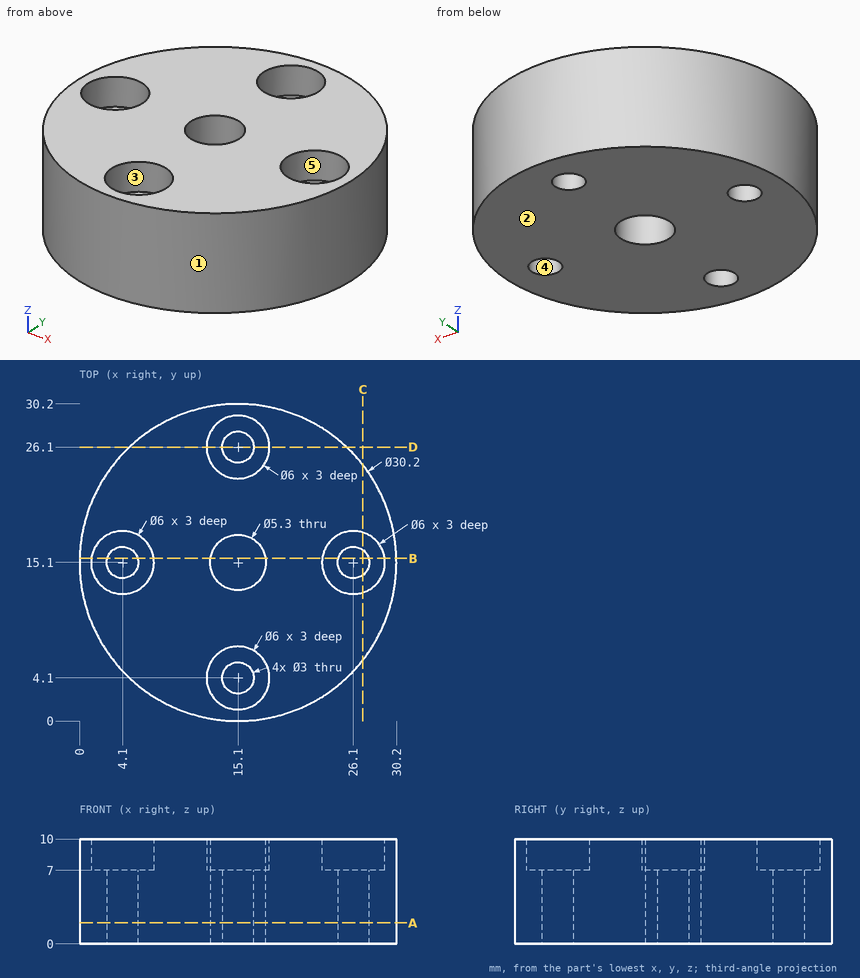
Study the drawing (mm; zero at the part's minimum x, y, z) and answer. A direction names the side the tool comes from. Round coordinates to 2 decimals unless told otherwise and drop trailing zeros. Loops run counter-clockwise (first coordinate to the right, second up) from the corner with the lowest first, then second, coordinate; pieces in that order, holes last. Notation, with made-up numbers: M 84,1.5 L 112,1.5 A21 cw 112,7.5 Z; hole C 65,86.25 d4. An arc over 180 degrees is marked long. One line per question, with ' | ' between items.
Q1. Find section B-B, the plane y = 15.5. Give the vertices of the cut face in (x, z).
Conclusion:
outline: M 0.01,0 L 2.65,0 L 2.65,7 L 1.13,7 L 1.13,10 L 0.01,10 Z; M 5.55,0 L 12.48,0 L 12.48,10 L 7.07,10 L 7.07,7 L 5.55,7 Z; M 17.72,0 L 24.65,0 L 24.65,7 L 23.13,7 L 23.13,10 L 17.72,10 Z; M 27.55,0 L 30.19,0 L 30.19,10 L 29.07,10 L 29.07,7 L 27.55,7 Z
Q2. Find section D-D, the plane y = 26.1. Give the vertices of the cut face in (x, z).
Conclusion:
outline: M 4.76,0 L 13.6,0 L 13.6,7 L 12.1,7 L 12.1,10 L 4.76,10 Z; M 16.6,0 L 25.44,0 L 25.44,10 L 18.1,10 L 18.1,7 L 16.6,7 Z
Q3. A tool of negligible diameter and unlimited length cuts with its end or side. For the marked faces 4 and 5, from which of +Z, -Z, +X, -X, +Y, -Y can it reach the whole face along a straight path? Write none if from no direction.
Conclusion:
face 4: +Z, -Z | face 5: +Z
Q4. Consider line 1 along Y through (x, z) = (15.1, 1.5); line 2 along Z through (x, y) = (13.5, 2); line 3 along Y through (x, z) = (25, 4.5). Determine where each line is inside the solid, lowest interval first. Write a range as from..to.
Conclusion:
line 1: y = 0..2.6, 5.6..12.45, 17.75..24.6, 27.6..30.2 | line 2: z = 0..7 | line 3: y = 3.7..14.08, 16.12..26.5
Q5. Find section C-C, the plane x = 27. Give the vertices of the cut face in (y, z), then the cut area to 3 significant figures.
Conclusion:
outline: M 5.8,0 L 13.9,0 L 13.9,7 L 12.24,7 L 12.24,10 L 5.8,10 Z; M 16.3,0 L 24.4,0 L 24.4,10 L 17.96,10 L 17.96,7 L 16.3,7 Z | area: 152 mm2
Q6. The mould has two halves that part along Y. Classify the marked faces 1, 2 and 3: +Y half, -Y half, draft (parallel to the pull), parting line (faces both ways), or undercut.
Conclusion:
face 1: parting line | face 2: draft | face 3: undercut
Q7. Find section A-A, the plane z = 2. Give the vertices of the cut face in (x, y), then the cut area to 3 significant figures.
Conclusion:
outline: C 15.1,15.1 d30.2; hole C 4.1,15.1 d3; hole C 15.1,15.1 d5.3; hole C 15.1,4.1 d3; hole C 15.1,26.1 d3; hole C 26.1,15.1 d3 | area: 666 mm2
Q8. Each of these flat-tipped pins is pushed along its axis until it touches: pin 1 Ø4 at (x, y) = (15.1, 4.1) entering from +Z; pin 2 Ø6 at (y, z) = (10.5, 6.5) entering from -X (3 decimals); pin 3 Ø1.5 at (x, z) = (17.5, 4.5) entering from +Y. Where does it stop, or does it pass through?
Conclusion:
pin 1: stops at z = 7 | pin 2: stops at x = 0.085 | pin 3: stops at y = 30.11
